Source: CAD feature listing. Evaluate the final solid. Frame: model axes, mm. Face numbers are marked on the shaded views. A direction names the side the tool comes from. Give positions to 0.01 mm unless a question says otherwise; leave off trailing zeros. Write each loop counter-clockwise with the first axis right and the second up, starting at its lowest first coordinate (ties: lowest second). Pieces come first, ordered by that corner, then holes. Notation, with made-up numbers: (48.25, 53.5) -> (99.25, 53.5) arc R16 cw to (99.25, 80.5) -> close; hole circle Ø10 at (75, 1). An arc over 180 degrees is marked (long way). Answer as a JSON object with one key per item and string values. Group by question number.
Item 1: Section query B-B on x = 2.25. Return the cut outline in (y, z).
Item 2: Section query D-D on y = 2.75. Return the cut outline in (x, z).
Item 3: Access query for the marked faces 1, 2 and 3. Directions: +Z, -Z, +X, -X, +Y, -Y. A direction counts if a zero-diameter tool reaches every point of the face in a straight line with its end or side. Return the directions, or none.
Item 4: Ray query, probe 1 along Z at (x, y) = (3, -1); probe 2 along Z at (x, y) = (0, 2); probe 3 along Y at (x, z) = (0, 2.75). Return the intervals inside material, ascending. Write a range as from..to.
Item 5: First-contact query: pin 1 Ø4 at (y, z) = (2.5, 7.5) entering from +X; pin 2 Ø3 at (x, z) = (2, 8) entering from -Y; pin 3 Ø4 at (x, y) = (-0.5, -0.5) entering from +Z. Flat tips, straight axial feed; report the tip coordinate or a pass-through.
Item 6: Section query A-A on y = 0. Return the cut outline in (x, z), plus the area to 3 significant figures.
Item 7: Section query C-C on z = 11. Return the cut outline in (x, y).
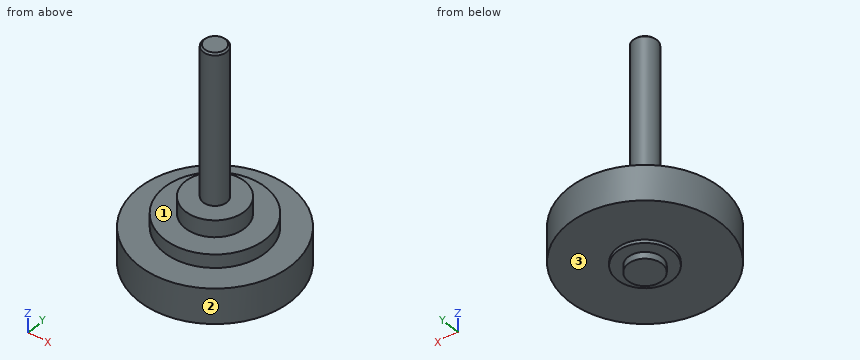
Autodesk Inventor part; units mm, degrees
ref_plane "YZ Plane" through (0, 0, 0) normal (1, 0, 0) x (0, 1, 0)
ref_plane "XZ Plane" through (0, 0, 0) normal (0, 1, 0) x (-1, 0, 0)
ref_plane "XY Plane" through (0, 0, 0) normal (0, 0, 1) x (1, 0, 0)
sketch "Эскиз1" plane through (0, 0, 0) normal (1, 0, 0) x (0, 1, 0)
  line L0 (0, 13.5) -> (0.7, 13.5)
  line L1 (0.7, 13.5) -> (0.7, 4.5)
  line L2 (0.7, 4.5) -> (1.75, 4.5)
  line L3 (1.75, 4.5) -> (1.75, 3.5)
  line L4 (1.75, 3.5) -> (3, 3.5)
  line L5 (3, 3.5) -> (3, 2.7)
  line L6 (3, 2.7) -> (4.5, 2.7)
  line L7 (4.5, 2.7) -> (4.5, 0.6)
  line L8 (0, 0) -> (0, 13.5)
  line L9 (1.6477, 0.4) -> (1, 0.4)
  line L10 (1, 0.4) -> (1, 0)
  line L11 (1, 0) -> (0, 0)
  line L12 (0, -2.7) -> (0, 16.2)
  line L13 (4.5, 0.6) -> (1.6477, 0.6)
  line L14 (1.6477, 0.6) -> (1.6477, 0.4)
  dimension "d0" = 1.4
  dimension "d1" = 13.5
  dimension "d2" = 9
  dimension "d3" = 2
  dimension "d4" = 0.4
  dimension "d5" = 0.2
  dimension "d6" = 9
  dimension "d7" = 1
  dimension "d8" = 0.8
  dimension "d9" = 3.5
  dimension "d10" = 6
revolve "Вращение1" add sketch "Эскиз1" angle 360 about axis through (0, 0, -10) along (0, 0, 1)
chamfer "Фаска1" distance 0.1 angle 45 1 edges at (0, -0.7, 13.5)
properties part number "Вал последний с чем то" material "Латунь, мягкая, желтая"
Worked answers:
{
 "1": {"outline": "(-3.9, 0.6) -> (3.9, 0.6) -> (3.9, 2.7) -> (1.98, 2.7) -> (1.98, 3.5) -> (-1.98, 3.5) -> (-1.98, 2.7) -> (-3.9, 2.7) -> close"},
 "2": {"outline": "(-3.56, 0.6) -> (3.56, 0.6) -> (3.56, 2.7) -> (1.2, 2.7) -> (1.2, 3.5) -> (-1.2, 3.5) -> (-1.2, 2.7) -> (-3.56, 2.7) -> close"},
 "3": {"face 1": "+Z", "face 2": "+Z, -Z", "face 3": "-Z"},
 "4": {"probe 1": "0.6..2.7", "probe 2": "0.6..3.5", "probe 3": "-3..3"},
 "5": {"pin 1": "x = 0.49", "pin 2": "y = -0.49", "pin 3": "z = 13.5"},
 "6": {"outline": "(-4.5, 0.6) -> (-1.65, 0.6) -> (-1.65, 0.4) -> (-1, 0.4) -> (-1, 0) -> (1, 0) -> (1, 0.4) -> (1.65, 0.4) -> (1.65, 0.6) -> (4.5, 0.6) -> (4.5, 2.7) -> (3, 2.7) -> (3, 3.5) -> (1.75, 3.5) -> (1.75, 4.5) -> (0.7, 4.5) -> (0.7, 13.4) -> (0.6, 13.5) -> (-0.6, 13.5) -> (-0.7, 13.4) -> (-0.7, 4.5) -> (-1.75, 4.5) -> (-1.75, 3.5) -> (-3, 3.5) -> (-3, 2.7) -> (-4.5, 2.7) -> close", "area": "41.2 mm^2"},
 "7": {"outline": "circle Ø1.4 at (0, 0)"}
}
